Autodesk Inventor part; units mm, degrees
ref_plane "YZ Plane" through (0, 0, 0) normal (1, 0, 0) x (0, 1, 0)
ref_plane "XZ Plane" through (0, 0, 0) normal (0, 1, 0) x (-1, 0, 0)
ref_plane "XY Plane" through (0, 0, 0) normal (0, 0, 1) x (1, 0, 0)
sketch "Sketch1" plane through (0, 0, 0) normal (0, 0, 1) x (1, 0, 0)
  line L0 (0, 0) -> (0, 125)
  dimension "d0" = 125
sketch "Sketch2" plane through (0, 0, 0) normal (0, 1, 0) x (-1, 0, 0)
  circle A0 centre (0, 0) radius 15
  dimension "d3" = 30
sweep "Sweep1" add profiles "Sketch2" path "Sketch1"
sketch "Sketch4" plane through (0, 0, 0) normal (1, 0, 0) x (0, 1, 0)
  line L0 (0, 17.5) -> (0, -17.5) construction
  line L1 (10, 17.5) -> (10, -17.5)
  line L2 (-10, -17.5) -> (-10, 17.5)
  arc A0 (10, 17.5) -> (-10, 17.5) centre (0, 17.5) ccw
  arc A1 (-10, -17.5) -> (10, -17.5) centre (0, -17.5) ccw
  line L3 (-10, 0) -> (10, 0)
  point P0 (0, 0)
  dimension "d9" = 35
  dimension "d10" = 10
revolve "Revolution1" add sketch "Sketch4" angle 360 about axis through (0, -10, 0) along (0, 1, 0) contours L1 L3 L2 A0
sketch "Sketch5" plane through (0, 0, 0) normal (0, 0, 1) x (1, 0, 0)
  line L0 (-30, 125) -> (30, 125)
  line L1 (30, 125) -> (30, 205)
  line L2 (30, 205) -> (-30, 205)
  line L3 (-30, 205) -> (-30, 125)
  circle A0 centre (0, 175) radius 12.5
  line L4 (0, 0) -> (0, 125) construction
  line L5 (0, 175) -> (0, 125)
  dimension "d12" = 175
  dimension "d13" = 25
  dimension "d14" = 60
  dimension "d15" = 30
extrude "Extrusion1" add sketch "Sketch5" along normal mid plane 80
sketch "Sketch7" plane through (-30, 125, 40) normal (-1, 0, 0) x (0, 0, 1)
  line L0 (-80, 80) -> (0, 80) construction
  line L1 (-65, 80) -> (-15, 80)
  line L2 (-15, 80) -> (-15, 20)
  line L3 (-15, 20) -> (-65, 20)
  line L4 (-65, 20) -> (-65, 80)
  line L5 (-80, 37.5) -> (-80, 62.5) construction
  line L6 (0, 62.5) -> (0, 37.5) construction
  line L7 (-80, 0) -> (-80, 80) construction
  line L8 (-80, 50) -> (0, 50) construction
  line L9 (0, 80) -> (0, 0) construction
  line L10 (-40, 50) -> (-40, 0) construction
  point P0 (-40, -125)
  dimension "d18" = 30
  dimension "d19" = 50
  dimension "d20" = 25
  dimension "d21" = 175
fillet "Fillet1" radius 10 13 edges at (-30, 165, 40) (30, 165, 40) (-30, 165, -40) (30, 165, -40) (-30, 125, 0) (0, 125, -40) (0, 125, 40) (30, 125, 0) (15, 125, 0) (-30, 205, 0) (0, 205, 40) (30, 205, 0) (0, 205, -40)
extrude "Extrusion2" cut sketch "Sketch7" against normal through all
equation "\"d20\" = 0.5 * d19"
properties part number "Elo-Bola Longo"
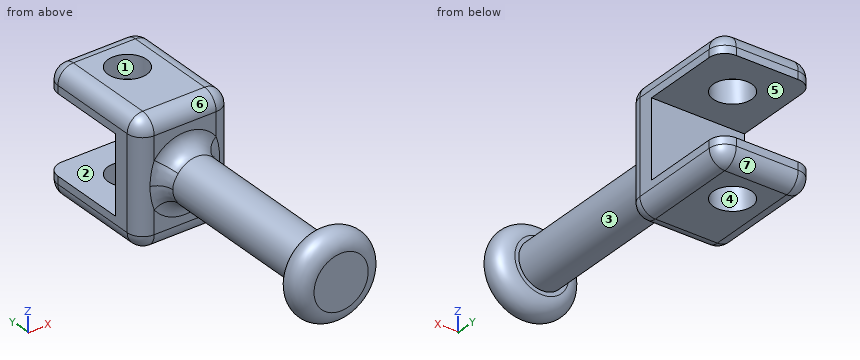
Geometry: final body of the model. Coordinates: model frame, mm. Face numbers are marked on the shaded views. A direction names the side the tool comes from. Give positions to 0.01 mm unless a question says otherwise; leave off trailing zeros. Order: outer loops, then holes, each group sorted by start corner. A loop starts at its lowest first (then second) coordinate and runs counter-clockwise, first axis right, second up. Notation, with made-up numbers: (41, 16.25) -> (84, 16.25) arc R16 ccw to (84, 47.25) -> close; hole circle Ø3 at (71, -30). An arc over 180 degrees is marked (long way). Answer as a JSON object with one key per item and string values.
Q1. Draft query along Z for the marked faces 4, 5, 6 and 7. Return one class per face: released by +Z, released by -Z, zero draft, split by the parting line, or undercut.
Entries:
{"face 4": "zero draft", "face 5": "undercut", "face 6": "released by +Z", "face 7": "released by -Z"}
Q2. Section B-B (x = 0). State how many separate pieces and enclosed holes the cut face has, plus the area to 3 significant figures.
Entries:
{"separate pieces": "3", "enclosed holes": "0", "area": "7,070 mm^2"}
Q3. Section A-A (y = 191.5). Output: boundary loops of the cut face in (x, z).
Entries:
{"outline": "(-30, -30) arc R10 ccw to (-20, -40) -> (20, -40) arc R10 ccw to (30, -30) -> (30, -25) -> (-30, -25) -> close; (-30, 25) -> (30, 25) -> (30, 30) arc R10 ccw to (20, 40) -> (-20, 40) arc R10 ccw to (-30, 30) -> close"}
Q4. Material intervals for probe 1 along Z at (x, y) = (-14, 187); probe 2 along X at (y, z) = (89.5, -9); probe 3 along Y at (x, z) = (-2, 3), sorted ascending.
Entries:
{"probe 1": "z = -40 to -25, 25 to 40", "probe 2": "x = -12 to 12", "probe 3": "y = -10 to 145"}
Q5. First-contact query: pin 1 (4 mm diameter, centred on x = -18, z = -13, fed in from +Y); pin 2 (16.5 mm diameter, centred on x = 5, z = 19, fed in from -Y); pin 3 (12 mm diameter, centred on x = -19.5, y = 68.5, fed in from -Z); pin 4 (1.5 mm diameter, centred on x = -22, y = 172.5, fed in from -Z). Flat tips, straight axial feed; report the tip coordinate or a pass-through.
Entries:
{"pin 1": "stops at y = 145", "pin 2": "stops at y = -10", "pin 3": "stops at z = -6.54", "pin 4": "stops at z = -39.92"}
Q6. Access query for the marked faces 1, 2 and 3. Directions: +Z, -Z, +X, -X, +Y, -Y. A direction counts if a zero-diameter tool reaches every point of the face in a straight line with its end or side. Return the directions, or none.
Entries:
{"face 1": "+Z, -Z", "face 2": "+X, -X, +Y", "face 3": "none"}
